Autodesk Inventor part; units mm, degrees
ref_plane "YZ Plane" through (0, 0, 0) normal (1, 0, 0) x (0, 1, 0)
ref_plane "XZ Plane" through (0, 0, 0) normal (0, 1, 0) x (-1, 0, 0)
ref_plane "XY Plane" through (0, 0, 0) normal (0, 0, 1) x (1, 0, 0)
ref_plane "Work Plane1" through (0, 0, 0) normal (0, 0, -1) x (-1, 0, 0)
sketch "Sketch3" plane through (0, 0, 0) normal (0, 0, -1) x (-1, 0, 0)
  circle A0 centre (0, 0) radius 11
  line L0 (-15.4, 0) -> (15.4, 0)
  dimension "d19" = 22
extrude "Extrusion3" add sketch "Sketch3" against normal blind 3.6
sketch "Sketch4" plane through (0, 0, 3.6) normal (0, 0, 1) x (1, 0, 0)
  arc A0 (10.6524, -2.5) -> (10.6524, 2.5) centre (0, 0) ccw
  line L0 (-16.2075, 0) -> (20.2449, 0)
  line L1 (15, 0) -> (15, 1.5)
  arc A1 (15, 1.5) -> (10.6524, 2.5) centre (9.5012, -12.4558) ccw
  line L2 (15, 0) -> (15, -1.5)
  arc A2 (10.6524, -2.5) -> (15, -1.5) centre (9.5012, 12.4558) ccw
  dimension "d22" = 1.5
  dimension "d23" = 2.5
  dimension "d24" = 15
  dimension "d25" = 15
extrude "Extrusion4" add sketch "Sketch4" against normal blind 3.6
sketch "Sketch2" plane through (0, 0, 0) normal (0, 0, -1) x (-1, 0, 0)
  line L0 (-9.8, -2.6) -> (-6, -2.6)
  line L1 (-6, -2.6) -> (-6, 2.6)
  line L2 (-6, 2.6) -> (-9.8, 2.6)
  line L3 (-9.8, 2.6) -> (-9.8, -2.6)
  line L4 (-9.8, -2.6) -> (-6, 2.6) construction
  line L5 (-6, -2.6) -> (-9.8, 2.6) construction
  line L6 (0, -27.5637) -> (0, 32.5752)
  line L7 (9.8, -2.6) -> (6, -2.6)
  line L8 (6, -2.6) -> (6, 2.6)
  line L9 (6, 2.6) -> (9.8, 2.6)
  line L10 (9.8, 2.6) -> (9.8, -2.6)
  line L11 (9.8, -2.6) -> (6, 2.6) construction
  line L12 (6, -2.6) -> (9.8, 2.6) construction
  point P0 (-7.9, 0)
  point P1 (7.9, 0)
  point P2 (0, 0)
  dimension "d11" = 3.8
  dimension "d12" = 5.2
  dimension "d31" = 6
  dimension "d32" = 0
extrude "Extrusion2" cut sketch "Sketch2" against normal blind 3.6
pattern_circular "Circular Pattern1" count 8 over 360 about axis through (0, 0, 0) along (0, 0, 1) of "Extrusion4"
properties part number "tandwiel(ja)"
Model file for the job. Use its own axes, mm. A direction names the side the tool comes from. Give positions to 0.01 mm unless a question says otherwise; leave off trailing zeros. Write each loop counter-clockwise with the first axis right and the second up, starting at its lowest first coordinate (ties: lowest second). Pieces come first, ordered by that corner, then holes. Notation, with made-up numbers: (89.25, -13.75) -> (147.25, -13.75) arc R16 cw to (147.25, 3.25) -> close; hole circle Ø8 at (-25.5, -38.75). An arc over 180 degrees is marked (long way). Use CSV: the item, a comma, the result in double quotes. Start each with the question number.
1) Cut at A-A on z = 1.65. Count the separate pieces of the cut face and the enclosed holes in it, plus the area to 3 significant figures.
2) Pin check, flat tip, straight feed: P1, Ø1.8, axis at x = 8.5, z = 1, coming from the +Y side. Stop position of the tip, or through.
3) Cut at C-C on x = -12.5. List the corners of the cut face in (y, z), plus the area to 3 significant figures.
4) Two-plate mould, pull along X, no slides. Class faces 6 (the flat face through (-8, 2.6, 2)), 7 (the cylindrical face through (10.66, -7.62, 1.83)), 8 (the flat face through (-15, 0, 2)), 9 (the cylindrical face through (2.15, -12.92, 1.83)): released by +X, released by -X, zero draft, split by the parting line, or undercut.
5) Drill centre lines: L1, parallel to X at y = -10, z = 0.4; L2, parallel to Y at x = -6.5, z = 3.1; L3, parallel to X at y = -5, z = 1.2. Where is each one in solid material? Low to high.
6) Tool access for faces 1 (the cylindrical face through (10.625, 7.566, 1.825)), 2 (the cylindrical face through (7.62, 10.66, 1.83)), 3 (the flat face through (9.8, 0, 2)), 4 (the cylindrical face through (-10.625, -7.566, 1.825)), 5 (the cylindrical face through (-4.19, -10.17, 1.77)): list every direction of +Z, -Z, +X, -X, +Y, -Y with a clear straight run to the whole face (end or side of a thin tool).
7) Cut at B-B on y = -3. List the corners of the cut face in (x, z), plus the area to 3 significant figures.
Final values:
1,separate pieces,"1"
1,enclosed holes,"2"
1,area,"478 mm2"
2,P1,"stops at y = 11.6"
3,outline,"(-2.24, 0) -> (2.24, 0) -> (2.24, 3.6) -> (-2.24, 3.6) -> close"
3,area,"16.1 mm2"
4,face 6,"undercut"
4,face 7,"released by +X"
4,face 8,"released by -X"
4,face 9,"undercut"
5,L1,"x = -11.21 to -6.65, -4.58 to 4.58, 6.65 to 11.21"
5,L2,"y = -9.89 to -2.6, 2.6 to 9.89"
5,L3,"x = -9.8 to 9.8"
6,face 1,"+Z, -Z, +X"
6,face 2,"+Z, -Z, +Y"
6,face 3,"+Z, -Z"
6,face 4,"+Z, -Z, -X"
6,face 5,"+Z, -Z, -Y"
7,outline,"(-10.58, 0) -> (10.58, 0) -> (10.58, 3.6) -> (-10.58, 3.6) -> close"
7,area,"76.2 mm2"
